Input: dimensioned drawing with shaded views. Units: mm. Origin: part minimum x, y, z. A direction names the side the tool comes from. Coordinates: 2 decimals unless noted, no trailing zeros. Loops run counter-clockwise (first coordinate to the right, second up) from the corner with the lowest first, then second, coordinate; pieces in that order, holes last.
(1) Mould query, pull axis Y, two halves, no side actions, for the marked faces 1, 2, 3 and 4. Classes: released by +Y, released by -Y, zero draft, split by the parting line, or undercut.
(2) Section C-C, the plane y = 56.5. Return loops of the section in (x, z).
(3) Set-up query: the marked faces 5 and 6. Return all of +Z, -Z, +X, -X, +Y, -Y with unobstructed straight access to the full face (end or side cutting, diameter ignored); none if empty.
(4) Section D-D, the plane x = 21. Return loops of the section in (y, z).
(5) Line query: L1, parallel to Y at x = 34, z = 60; L2, parallel to Y at x = 34, z = 67.75; L3, parallel to Y at x = 54.5, z = 18. Output: solid intervals per line, ascending.
(6) Contact query for flat-ended pins moving along their axis: P1, Ø6, axis at x = 34, y = 61, coming from the +Z side; P2, Ø3.5, axis at x = 34, y = 61.5, coming from the +Z side; P3, Ø6, axis at y = 51, z = 28, coming from the -X side. Output: stop coordinate, or through.
(7) Section B-B, the plane z = 63.5. Return loops of the section in (x, y).
(8) Section A-A, the plane x = 34. Return loops of the section in (y, z), then the cut area to 3 significant figures.
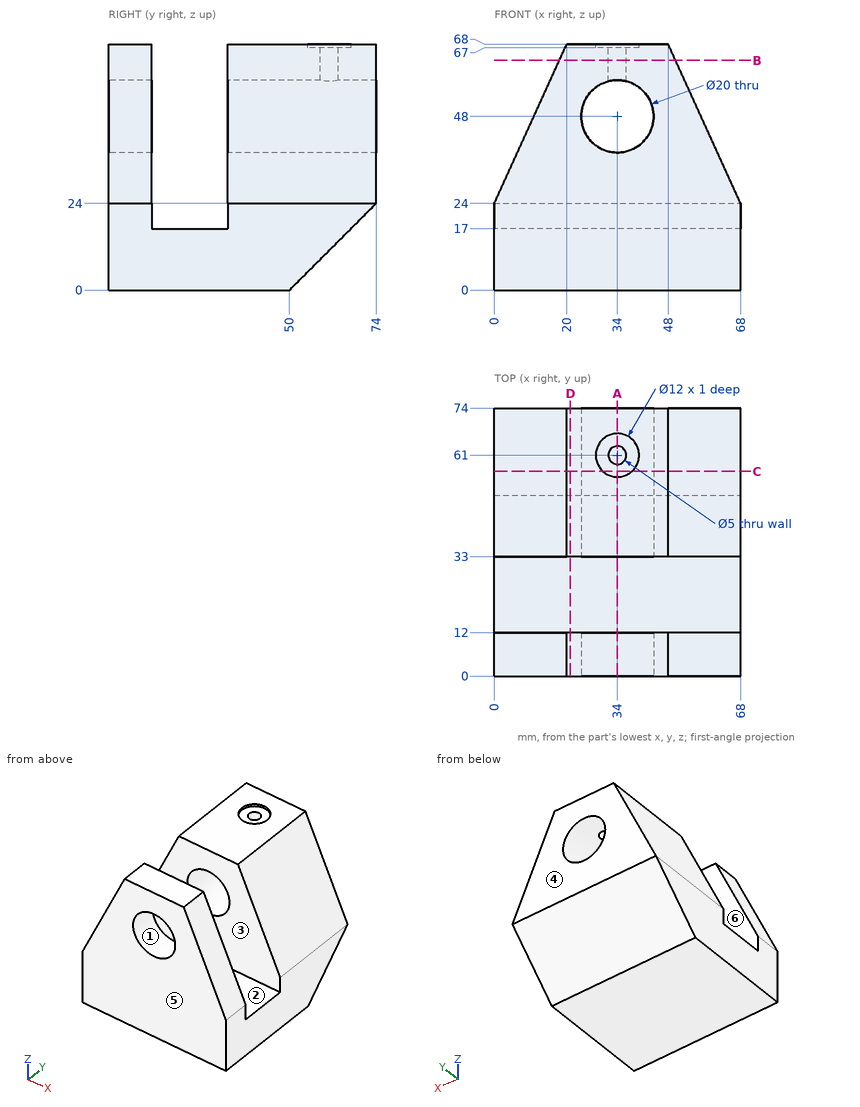
Report:
1. face 1: zero draft
1. face 2: undercut
1. face 3: undercut
1. face 4: released by +Y
2. outline: (0, 6.5) - (68, 6.5) - (68, 24) - (48, 68) - (37.97, 68) - (37.97, 67) - (30.03, 67) - (30.03, 68) - (20, 68) - (0, 24) - close; hole circle Ø20 at (34, 48)
3. face 5: +Z, -Z, +X, -X, -Y
3. face 6: +Z, +X, -X
4. outline: (0, 0) - (50, 0) - (74, 24) - (74, 68) - (33, 68) - (33, 17) - (12, 17) - (12, 68) - (0, 68) - close
5. L1: y = 0 to 12, 33 to 58.5, 63.5 to 74
5. L2: y = 0 to 12, 33 to 55, 67 to 74
5. L3: y = 0 to 12, 33 to 68
6. P1: stops at z = 67
6. P2: stops at z = 38.15
6. P3: stops at x = 0.45
7. outline: (17.95, 0) - (50.05, 0) - (50.05, 12) - (17.95, 12) - close; (17.95, 33) - (50.05, 33) - (50.05, 74) - (17.95, 74) - close; hole circle Ø5 at (34, 61)
8. outline: (0, 0) - (50, 0) - (74, 24) - (74, 38) - (33, 38) - (33, 17) - (12, 17) - (12, 38) - (0, 38) - close; (0, 58) - (12, 58) - (12, 68) - (0, 68) - close; (33, 58) - (58.5, 58) - (58.5, 67) - (55, 67) - (55, 68) - (33, 68) - close; (63.5, 58) - (74, 58) - (74, 68) - (67, 68) - (67, 67) - (63.5, 67) - close
8. area: 2,560 mm2
